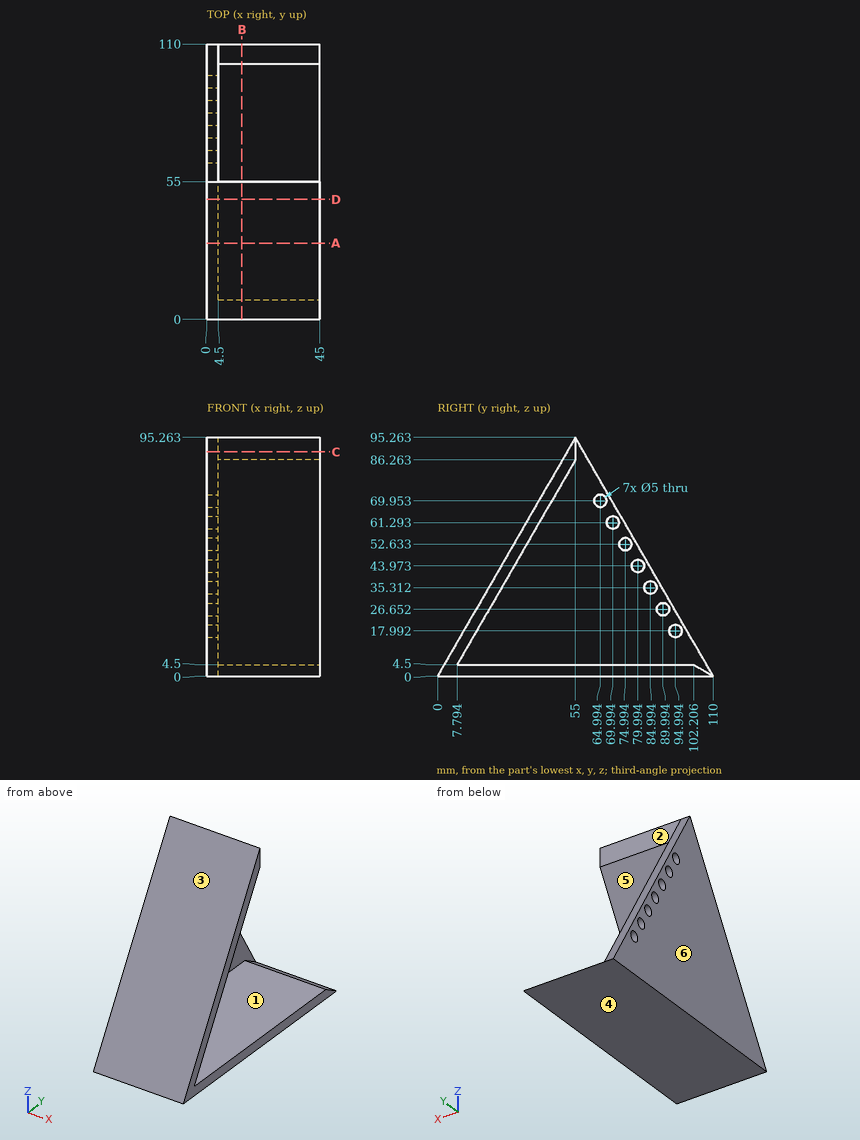
Geometry: see drawing. Coordinates: mm, zero at the bounding-box minimum. A direction names the side the tool comes from. Coordinates: 2 decimals unless noted, no trailing zeros. Loops run counter-clockwise (first coordinate to the right, second up) from the corner with the lowest first, then second, coordinate; pieces in that order, holes last. Notation, with made-up numbers: (80.25, 83) - (113.25, 83) arc R18 ccw to (113.25, 91) - close; hole circle Ø6 at (8, 7). An arc over 180 degrees is marked (long way). Answer in a Markdown table with one row per item.
(1) Cut plane B-B on x = 14. Output: boundary loops of the cut face in (y, z) (1 decimal), plus the area to 3 significant figures.
Model answer:
| item | result |
|---|---|
| outline | (0, 0) - (110, 0) - (102.2, 4.5) - (7.8, 4.5) - (55, 86.3) - (55, 95.3) - close |
| area | 920 mm² |
(2) Mould query, pull axis Z, two halves, no side actions, for the marked faces 4, 5 and 6. Classes: pulls with the +Z half, pulls with the -Z half, needs draft (parallel to the pull), parting line crosses it, or undercut.
Model answer:
| item | result |
|---|---|
| face 4 | pulls with the -Z half |
| face 5 | undercut |
| face 6 | needs draft |
(3) Cut plane A-A on y = 30.5. Output: boundary loops of the cut face in (x, z).
Model answer:
| item | result |
|---|---|
| outline | (0, 0) - (45, 0) - (45, 4.5) - (4.5, 4.5) - (4.5, 43.83) - (45, 43.83) - (45, 52.83) - (0, 52.83) - close |
(4) Cut plane D-D on y = 48. Output: boundary loops of the cut face in (x, z), plus the area to 3 significant figures.
Model answer:
| item | result |
|---|---|
| outline | (0, 0) - (45, 0) - (45, 4.5) - (4.5, 4.5) - (4.5, 74.14) - (45, 74.14) - (45, 83.14) - (0, 83.14) - close |
| area | 921 mm² |
(5) Cut plane C-C on z = 89.5. Output: boundary loops of the cut face in (x, y).
Model answer:
| item | result |
|---|---|
| outline | (0, 51.67) - (45, 51.67) - (45, 55) - (4.5, 55) - (4.5, 58.33) - (0, 58.33) - close |
(6) Pin query (flat end, axial travel): P1, Ø6.5, axis at y = 64.99, z = 69.95, coming from the -X side; P2, Ø10, axis at x = 23, y = 90, coming from the +Z side; P3, Ø6, axis at x = 40.5, y = 15.5, coming from the +Z side (1 decimal); P4, Ø2.5, axis at x = 34.5, z = 92.5, coming from the +Y side. Return the tip coordinate at first contact, or that it passes through.
Model answer:
| item | result |
|---|---|
| P1 | stops at x = 0 |
| P2 | stops at z = 4.5 |
| P3 | stops at z = 32 |
| P4 | stops at y = 55 |
(7) Material intervals for L1, parallel to X at y = 90, z = 31.5; L2, parallel to Z at x = 42, y = 15, sorted ascending. Write a range as from..to.
Model answer:
| item | result |
|---|---|
| L1 | x = 0..4.5 |
| L2 | z = 0..4.5, 16.98..25.98 |
(8) Set-up query: the marked faces 1, 2 and 3. Return all of +Z, -Z, +X, -X, +Y, -Y with unobstructed straight access to the full face (end or side cutting, diameter ignored); none if empty.
Model answer:
| item | result |
|---|---|
| face 1 | +X, +Y |
| face 2 | +Z, +X, +Y |
| face 3 | +Z, +X, -X, -Y |
